Geometry check sheet. Reference: the model listing, model coordinates, mm. Face numbers are marked on the shaded views. A direction names the side the tool comes from. Coordinates: 2 decimals unless noted, no trailing zeros. Loops run counter-clockwise (first coordinate to the right, second up) from the corner with the lowest first, then second, coordinate; pieces in that order, holes last.
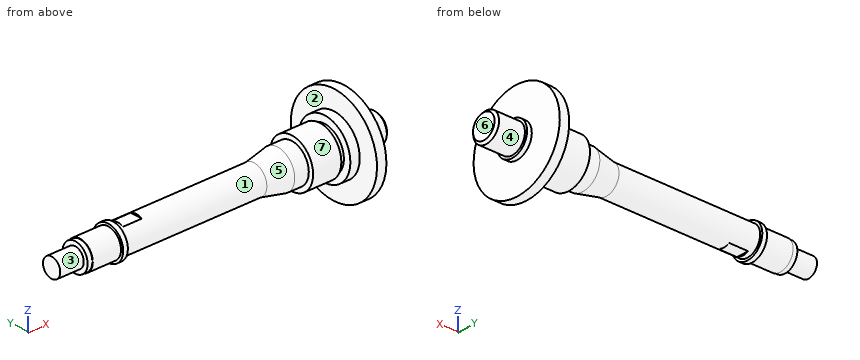
from build123d import *

# Parameters (mm, degrees)
SKETCH_1_R          = 10
EXTRUDE_1_DEPTH     = 2
SKETCH_2_R          = 3.5
EXTRUDE_2_DEPTH     = 1
SKETCH_3_R          = 6
EXTRUDE_3_DEPTH     = 9
SKETCH_4_R          = 4
EXTRUDE_4_DEPTH     = 3
SKETCH_5_R          = 3
EXTRUDE_5_DEPTH     = 6
EXTRUDE_START       = 35
SKETCH_6_R          = 3
EXTRUDE_6_DEPTH     = 35
EXTRUDE_START_2     = 1
SKETCH_7_R          = 3.5
EXTRUDE_7_DEPTH     = 1
EXTRUDE_START_3     = 9
SKETCH_8_R          = 3
EXTRUDE_8_DEPTH     = 9
SKETCH_9_R          = 2
EXTRUDE_9_DEPTH     = 3
CHAMFER_1_SIZE      = 0.5
SKETCH_11_W         = 4
SKETCH_11_H         = 0.3
CUT_EXTRUDE_2_DEPTH = 5
CUT_EXTRUDE_START   = 2
SKETCH_12_R         = 6
SKETCH_12_R_2       = 4.5
CUT_EXTRUDE_3_DEPTH = 1
CUT_EXTRUDE_START_2 = -6
SKETCH_13_R         = 6
SKETCH_13_R_2       = 5
CUT_EXTRUDE_4_DEPTH = 6
SKETCH_15_R         = 3
SKETCH_15_R_2       = 2.9
CUT_EXTRUDE_5_DEPTH = 3
SKETCH_16_R         = 2.9
SKETCH_16_R_2       = 2
CUT_EXTRUDE_8_DEPTH = 2


with BuildPart() as part:
    # 草图1 → 凸台-拉伸1 (new body)
    with BuildSketch(Plane(origin=(0, 0, 0), x_dir=(0, 0, -1), z_dir=(1, 0, 0))):
        Circle(SKETCH_1_R)
    extrude(amount=EXTRUDE_1_DEPTH)

    # 草图2 → 凸台-拉伸2 (add)
    with BuildSketch(Plane(origin=(2, 0, 0), x_dir=(0, 0, -1), z_dir=(1, 0, 0))):
        Circle(SKETCH_2_R)
    extrude(amount=EXTRUDE_2_DEPTH)

    # 草图3 → 凸台-拉伸3 (add)
    with BuildSketch(Plane.ZY):
        with Locations(Location((0, 0, 0), (0, 0, 180))):
            Circle(SKETCH_3_R)
    extrude(amount=EXTRUDE_3_DEPTH)

    # 草图4 → 凸台-拉伸4 (add)
    with BuildSketch(Plane.ZY.offset(9)):
        Circle(SKETCH_4_R)
    extrude(amount=EXTRUDE_4_DEPTH)

    # 草图5 → 凸台-拉伸5 (add)
    with BuildSketch(Plane(origin=(3, 0, 0), x_dir=(0, 0, -1), z_dir=(1, 0, 0))):
        Circle(SKETCH_5_R)
    extrude(amount=EXTRUDE_5_DEPTH)

    # 草图6 → 凸台-拉伸6 (add)
    with BuildSketch(Plane.ZY.offset(12).offset(EXTRUDE_START)):
        with Locations(Location((0, 0, 0), (0, 0, 180))):
            Circle(SKETCH_6_R)
    extrude(amount=-EXTRUDE_6_DEPTH)

    # 草图7 → 凸台-拉伸7 (add)
    with BuildSketch(Plane.ZY.offset(47).offset(EXTRUDE_START_2)):
        with Locations(Location((0, 0, 0), (0, 0, 180))):
            Circle(SKETCH_7_R)
    extrude(amount=-EXTRUDE_7_DEPTH)

    # 草图8 → 凸台-拉伸8 (add)
    with BuildSketch(Plane.ZY.offset(48).offset(EXTRUDE_START_3)):
        with Locations(Location((0, 0, 0), (0, 0, 180))):
            Circle(SKETCH_8_R)
    extrude(amount=-EXTRUDE_8_DEPTH)

    # 草图9 → 凸台-拉伸9 (add)
    with BuildSketch(Plane.ZY.offset(57)):
        Circle(SKETCH_9_R)
    extrude(amount=EXTRUDE_9_DEPTH)

    # 倒角1
    chamfer_1_edges = [part.edges().sort_by_distance(p)[0] for p in [
        (9, 0, 3),
    ]]
    chamfer(chamfer_1_edges, length=CHAMFER_1_SIZE)

    # 草图11 → 切除-拉伸2 (cut, symmetric)
    with BuildSketch(Plane(origin=(0, 0, 0), x_dir=(1, 0, 0), z_dir=(0, 1, 0))):
        with Locations((-44, 2.85)):
            Rectangle(SKETCH_11_W, SKETCH_11_H)
        with Locations((-44, -2.85)):
            Rectangle(SKETCH_11_W, SKETCH_11_H)
    extrude(amount=CUT_EXTRUDE_2_DEPTH, both=True, mode=Mode.SUBTRACT)

    # 草图12 → 切除-拉伸3 (cut)
    with BuildSketch(Plane.ZY.offset(CUT_EXTRUDE_START)):
        Circle(SKETCH_12_R)
        Circle(SKETCH_12_R_2, mode=Mode.SUBTRACT)
    extrude(amount=CUT_EXTRUDE_3_DEPTH, mode=Mode.SUBTRACT)

    # 草图13 → 切除-拉伸4 (cut)
    with BuildSketch(Plane.ZY.offset(9).offset(CUT_EXTRUDE_START_2)):
        with Locations(Location((0, 0, 0), (0, 0, 180))):
            Circle(SKETCH_13_R)
        Circle(SKETCH_13_R_2, mode=Mode.SUBTRACT)
    extrude(amount=CUT_EXTRUDE_4_DEPTH, mode=Mode.SUBTRACT)

    # 草图14 → 旋转1 (revolve)
    with BuildSketch(Plane.XY, mode=Mode.PRIVATE) as revolve_1_sk:
        Polygon((-12, 4), (-17, 3), (-12, 3), align=None)
    revolve(revolve_1_sk.sketch.rotate(Axis((-6.238584256, 0, 0), (-1, 0, 0)), 90), axis=Axis((-6.238584256, 0, 0), (-1, 0, 0)))

    # 草图15 → 切除-拉伸5 (cut)
    with BuildSketch(Plane.ZY.offset(57)):
        Circle(SKETCH_15_R)
        Circle(SKETCH_15_R_2, mode=Mode.SUBTRACT)
    extrude(amount=-CUT_EXTRUDE_5_DEPTH, mode=Mode.SUBTRACT)

    # 草图16 → 切除-拉伸8 (cut)
    with BuildSketch(Plane.ZY.offset(57)):
        Circle(SKETCH_16_R)
        Circle(SKETCH_16_R_2, mode=Mode.SUBTRACT)
    extrude(amount=-CUT_EXTRUDE_8_DEPTH, mode=Mode.SUBTRACT)


solid = part.part
(1) Scan lines: L1, parallel to X at y = -3.25, z = 3.25; L2, parallel to Z at x = 1, y = 0.25; L3, parallel to X at y = 7.5, z = -1.25. Record each from-to range of solid material in increasing order.
Findings:
L1: x = -9 to -3, -2 to 2
L2: z = -10 to 10
L3: x = 0 to 2
(2) Draft check along X on the marked faces 1, 2 and 3. Enter one of: +X half, -X half, draft (parallel to the pull), parting line (faces both ways), or undercut.
Findings:
face 1: undercut
face 2: -X half
face 3: draft
(3) Sectioned sample at A-A on x = -24.5. Record the cut outline in (y, z).
Findings:
outline: circle Ø6 at (0, 0)
(4) Access from +Z, -Z, +X, -X, +Y, -Y to the whole of each face (thin tool, end or side, straight path). Record for the marked faces 4, 5, 6 and 7.
Findings:
face 4: +X
face 5: none
face 6: +Z, -Z, +X, +Y, -Y
face 7: -X
(5) Gauge pin test, flat ends, axial feed: pin 1 Ø1.3 at (x, y) = (-43, 0.5) entering from -Z; pin 2 Ø12 at (x, y) = (-18.5, 5.5) entering from -Z; pin 3 Ø3 at (x, z) = (-37.5, -1.5) entering from -Y. Record the tip position at first contact, or that the pin passes through.
Findings:
pin 1: stops at z = -2.7
pin 2: stops at z = -3.35
pin 3: stops at y = -3
